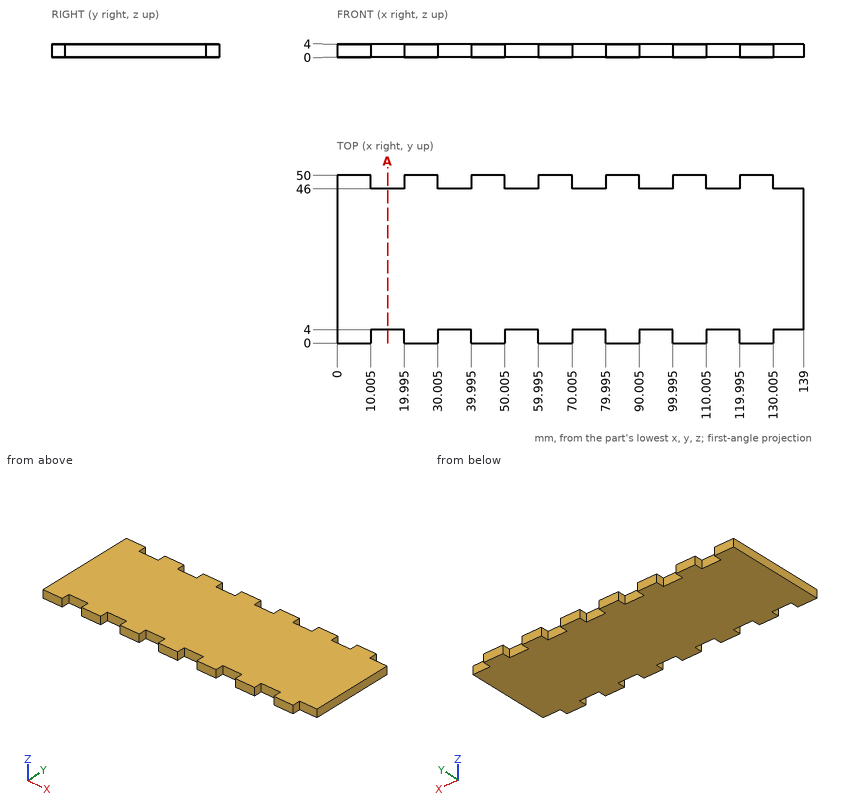
Can you work these out from the drawing? Everything is in mm from the part's minimum corner. Give positions to 0.01 mm unless a question says otherwise; leave off trailing zeros. Loops run counter-clockwise (first coordinate to the right, second up) from the corner with the lowest first, then second, coordinate; pieces in that order, holes last. Notation, with made-up numbers: (87.25, 9.25) -> (123.25, 9.25) arc R19 cw to (123.25, 43.25) -> close; hole circle Ø11 at (-7, 80). An arc over 180 degrees is marked (long way). Return JSON: item names as keys, results as strings.
Item 1: I need wall thicknesses on L1, parallel to Y at x = 131.5, z = 3.55. Which ranges of the line are inside material? Lowest first, please. Write a range as from..to.
Geometry results:
{"L1": "y = 4..46"}
Item 2: I'm going to push flat-ended pins straight in: pin 1 (1.2 mm diameter, centred on y = 47.5, z = 1.5, fed in from +X) (3 decimals); pin 2 (2 mm diameter, centred on x = 133.5, z = 1, fed in from +Y); pin 3 (3 mm diameter, centred on x = 100, y = 26.5, fed in from -Z); pin 4 (2 mm diameter, centred on x = 115.5, z = 1.5, fed in from -Y). Where does each tip first touch, or does it pass through?
Geometry results:
{"pin 1": "stops at x = 130.005", "pin 2": "stops at y = 46", "pin 3": "stops at z = 0", "pin 4": "stops at y = 4"}
Item 3: If we section it at A-A on x = 15: List the corners of the cut face in (y, z) for me.
Geometry results:
{"outline": "(4, 0) -> (46, 0) -> (46, 4) -> (4, 4) -> close"}
